The figure shows three views and two pictorial views of one solid part (mm, origin at its lowest corner). Answer the questions. A direction names the side the tool comes from. Give positions to 0.01 mm unless a question says otherwise; leave off trailing zeros. Order: outer loops, then holes, each group sorted by start corner. A loop starts at its lowest first (then second) coordinate and runs counter-clockwise, first axis right, second up. Notation, with made-up numbers: M 19.5,63 L 46.5,63 A32 ccw 46.5,101 Z; hole C -4.75,7.25 d5. An arc over 180 degrees is marked long. One line per item, written item: value.
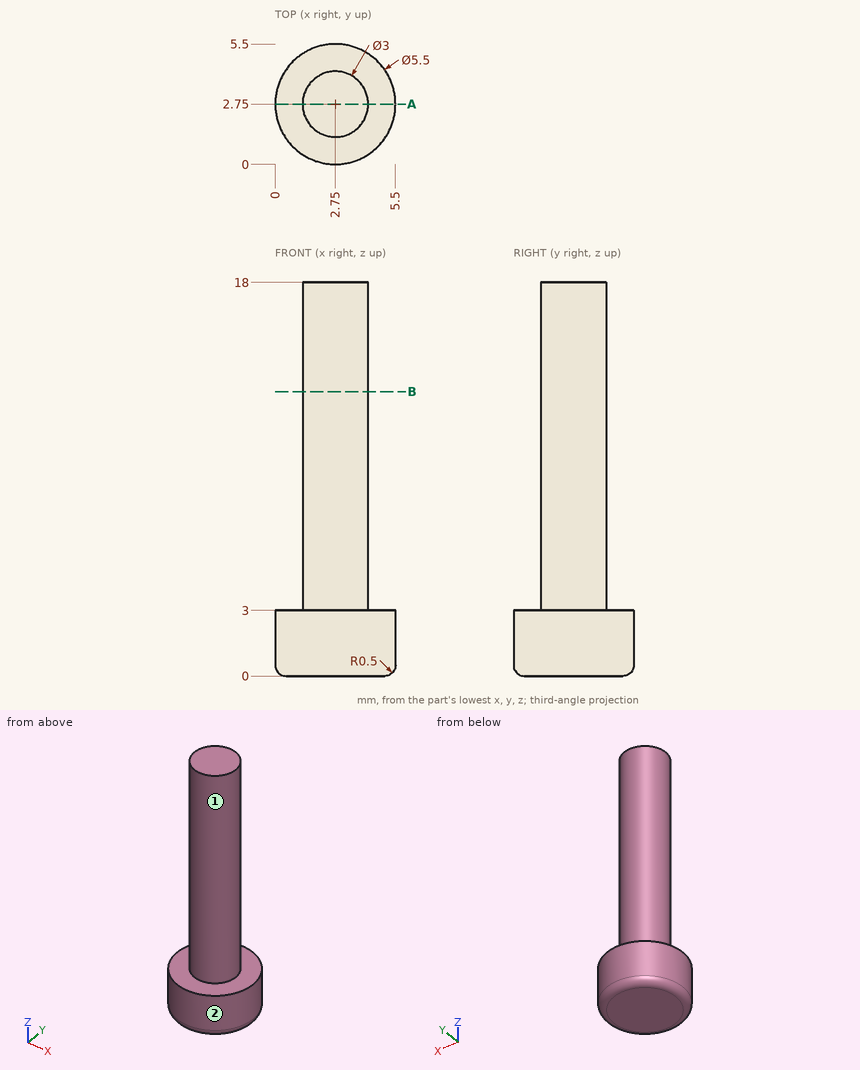
1) Find section B-B, the plane z = 13. Write down the section's boundary in (x, y).
Reported:
outline: C 2.75,2.75 d3
2) Consider probe 1 along Z at (x, y) = (1.9, 4.65); probe 2 along X at (y, z) = (2.5, 1); probe 3 along Y at (x, z) = (1.5, 12.25). Determine where each line is inside the solid, lowest interval first.
Reported:
probe 1: z = 0 to 3
probe 2: x = 0.01 to 5.49
probe 3: y = 1.92 to 3.58
3) Find section A-A, the plane y = 2.75. Write down the section's boundary in (x, z), plus the area to 3 significant figures.
Reported:
outline: M 0,0.5 A0.5 ccw 0.5,0 L 5,0 A0.5 ccw 5.5,0.5 L 5.5,3 L 4.25,3 L 4.25,18 L 1.25,18 L 1.25,3 L 0,3 Z
area: 61.4 mm^2
4) Which of the six approach directions +Z, -Z, +X, -X, +Y, -Y give full straight-line access (tool end or side, diameter ignored) to the marked faces 1 and 2?
Reported:
face 1: +Z
face 2: +Z, -Z
5) This flat-tipped pin is pushed along its axis until it touches: pin 1 Ø1 at (x, z) = (4.5, 4.5) entering from +Y. Where does it stop, or does it pass through?
Reported:
pin 1: stops at y = 3.58
